Here's how the part is built. I have some questions about the finished solid (model axes, mm). A direction names the side the tool comes from. Give positions to 0.01 mm unless a question says otherwise; leave off trailing zeros. Loops run counter-clockwise (first coordinate to the right, second up) from the corner with the lowest first, then second, coordinate; pieces in that order, holes last. Notation, with made-up numbers: M 6,26.5 L 58,26.5 A3 cw 58,30.5 Z; hole C -28,-28.5 d9. An arc over 180 degrees is marked long. Write item = value, one per line. Start each with the question number.
```python
from build123d import *

# Parameters (mm, degrees)
BOSS_EXTRUDE1_DEPTH = 19.05
CUT_EXTRUDE1_DEPTH  = 20.05


with BuildPart() as part:
    # Sketch1 → Boss-Extrude1 (new body)
    with BuildSketch(Plane.XY):
        Polygon((-65.216216216, 23.340540541), (-65.216216216, -52.859459459), (36.383783784, -52.859459459), (36.383783784, -27.459459459), (544.383783784, -27.459459459), (544.383783784, -2.059459459), (36.383783784, -2.059459459), (36.383783784, 23.340540541), align=None)
    extrude(amount=BOSS_EXTRUDE1_DEPTH)

    # Sketch2 → Cut-Extrude1 (cut, through all)
    with BuildSketch(Plane.XY.offset(19.05)):
        with BuildLine():
            Line((-12.037570257, -3.904520508), (-12.038141216, -1.524538483))
            Line((-12.038141216, -1.524538483), (-16.800641216, -1.524538483))
            Line((-16.800641216, -1.524538483), (-16.800641216, -3.905788483))
            ThreePointArc((-16.800641216, -3.905788483), (-14.413257962, -25.871959066), (-12.037570257, -3.904520508))
        make_face()
    extrude(amount=-CUT_EXTRUDE1_DEPTH, mode=Mode.SUBTRACT)


solid = part.part
```
Q1. If we section it at A-A, the plane z = 8: List the corners of the cut face in (x, y) for me (1 decimal), then the cut area to 3 significant figures.
Q2. Will these pins go through, and if not, where does the flat tip stop? pin 1 (10 mm diameter, centred on y = 3, z = 5.5, fed in from +X); pin 2 (10 mm diameter, centred on x = 242.5, z = 15.5, fed in from +Y); pin 3 (6 mm diameter, centred on x = 119, z = 9, fed in from -Y); pin 4 (1 mm diameter, centred on x = 325.5, y = -3.5, fed in from -Z).
Q3. If we section it at B-B, the plane y = -18: List the corners of the cut face in (x, z) for me.
Q4. If I drill on line 1 along X through (y, z) = (17.5, 14.5); line 2 along Y through (x, z) = (247, 15.25); line 3 along X through (y, z) = (-7, 15.5), over which ranges is the centre line in solid material (lowest first)?
Q5. If we section it at C-C, the plane x = 317: List the corners of the cut face in (y, z) for me.
Q6. If we section it at D-D, the plane y = 4.5: List the corners of the cut face in (x, z) for me.
Q7. On a 3-axis mill with a long thin cutter (end or side, diameter ignored), from which of +Z, -Z, +X, -X, +Y, -Y can I reach the whole of each face in a straight line? I mean faces 4 (the flat face through (36.384, 10, 9)), 5 (the flat face through (36.384, -40, 9)), 6 (the flat face through (-15, -52.859, 9)). Say none if no direction works.
Q8. We'd pull the mould along Y, two halves only. Please class faces 1 (the flat face through (168, -14, 19.05)), 2 (the cylindrical face through (-14.868, -25.863, 9.658)), 3 (the flat face through (-14, 23.341, 9)): pulls with the +Y half, pulls with the -Y half, needs draft (parallel to the pull), parting line crosses it, or undercut.
Resolved:
q1.outline = M -65.2,-52.9 L 36.4,-52.9 L 36.4,-27.5 L 544.4,-27.5 L 544.4,-2.1 L 36.4,-2.1 L 36.4,23.3 L -65.2,23.3 Z; hole M -16.8,-3.9 A11.1 ccw long -12,-3.9 L -12,-1.5 L -16.8,-1.5 Z
q1.area = 20,200 mm²
q2.pin_1 = 36.38
q2.pin_2 = -2.06
q2.pin_3 = -27.46
q2.pin_4 = 0
q3.outline = M -65.22,0 L -25.05,0 L -25.05,19.05 L -65.22,19.05 Z; M -3.79,0 L 544.38,0 L 544.38,19.05 L -3.79,19.05 Z
q4.line_1 = -65.22 to 36.38
q4.line_2 = -27.46 to -2.06
q4.line_3 = -65.22 to -22.37, -6.46 to 544.38
q5.outline = M -27.46,0 L -2.06,0 L -2.06,19.05 L -27.46,19.05 Z
q6.outline = M -65.22,0 L 36.38,0 L 36.38,19.05 L -65.22,19.05 Z
q7.face_4 = +Z, -Z, +X, +Y
q7.face_5 = +Z, -Z, +X, -Y
q7.face_6 = +Z, -Z, +X, -X, -Y
q8.face_1 = needs draft
q8.face_2 = undercut
q8.face_3 = pulls with the +Y half
